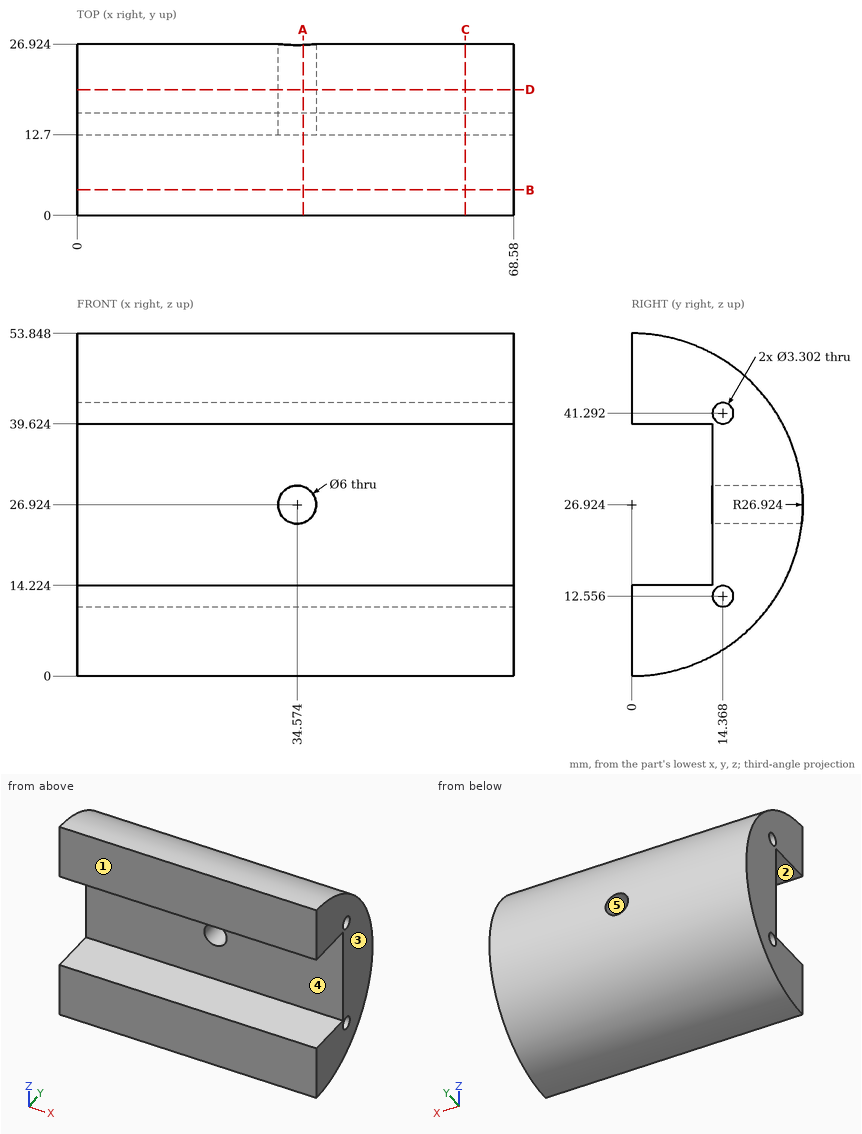
Job drawing, mm, ordinate dimensions from the low corner. One solid piece. A direction names the side the tool comes from. Coordinates: 2 decimals unless noted, no trailing zeros. Order: outer loops, then holes, each group sorted by start corner. A loop starts at its lowest first (then second) coordinate and runs counter-clockwise, first axis right, second up. Notation, with made-up numbers: (-15, -13.75) - (24, -13.75) arc R17 ccw to (24, 6.25) - close; hole circle Ø4 at (-38.75, 11). An arc over 180 degrees is marked (long way). Return JSON: item names as keys, results as strings. Group by question number.
1) Saw through at D-D, the plane y = 19.75. Write the cut outline in (x, z) (1 decimal), plus the area to 3 significant figures.
2) Saw through at A-A, the plane x = 35.5. Write the cut outline in (y, z) (1 decimal).
3) Flat gauge pins, fed straight in: P1, Ø1.5, axis at x = 50.5, y = 16.5, coming from the -Z side; P2, Ø2, axis at x = 37, z = 27.5, coming from the -Y side; P3, Ø1.5, axis at x = 17.5, y = 18.5, coming from the -Z side; P4, Ø10, axis at y = 5.5, z = 22, coming from the +X side. Where does each tip first touch, or does it go through?
4) Tool access for the marked faces 1 and 2: list every direction of +Z, -Z, +X, -X, +Y, -Y with a clear straight run to the whole face (end or side of a thin tool).
5) Mould opens along X. For the marked faces 3, 4 and 5 say: released by +X, released by -X, zero draft, split by the parting line, or undercut.
6) Saw through at B-B, the plane y = 4. Write the cut outline in (x, z), plus the area to 3 significant figures.
7) Probe line 1 (Z direction, x = 60, y = 14) (1 decimal); line 2 (X direction, y = 16, z = 25.5) (1 decimal); line 3 (Y direction, x = 52.5, z = 28). List the from-to ranges inside material, lowest first. Write a range as from..to.
8) Saw through at C-C, the plane x = 61. Write the cut outline in (y, z) (1 decimal), plus the area to 3 significant figures.
Values found:
{
 "1": {"outline": "(0, 8.6) - (68.6, 8.6) - (68.6, 45.2) - (0, 45.2) - close; hole circle Ø6 at (34.6, 26.9)", "area": "2,480 mm²"},
 "2": {"outline": "(0, 0) arc R26.9 ccw to (26.8, 24.1) - (12.7, 24.1) - (12.7, 14.2) - (0, 14.2) - close; (0, 39.6) - (12.7, 39.6) - (12.7, 29.8) - (26.8, 29.8) arc R26.9 ccw to (0, 53.8) - close; hole circle Ø3.3 at (14.4, 12.6); hole circle Ø3.3 at (14.4, 41.3)"},
 "3": {"P1": "stops at z = 5.09", "P2": "stops at y = 12.7", "P3": "stops at z = 6.68", "P4": "passes through"},
 "4": {"face 1": "+Z, -Z, +X, -X, -Y", "face 2": "+X, -X, -Y"},
 "5": {"face 3": "released by +X", "face 4": "zero draft", "face 5": "undercut"},
 "6": {"outline": "(0, 0.3) - (68.58, 0.3) - (68.58, 14.22) - (0, 14.22) - close; (0, 39.62) - (68.58, 39.62) - (68.58, 53.55) - (0, 53.55) - close", "area": "1,910 mm²"},
 "7": {"line 1": "z = 3.9..10.9, 14.2..39.7, 42.9..49.9", "line 2": "x = 0..31.9, 37.2..68.6", "line 3": "y = 12.7..26.9"},
 "8": {"outline": "(0, 0) arc R26.9 ccw to (0, 53.8) - (0, 39.6) - (12.7, 39.6) - (12.7, 14.2) - (0, 14.2) - close; hole circle Ø3.3 at (14.4, 12.6); hole circle Ø3.3 at (14.4, 41.3)", "area": "799 mm²"}
}
